```python
from build123d import *

# Parameters (mm, degrees)
SKETCH1_W           = 48.26
SKETCH1_H           = 17.78
BOSS_EXTRUDE1_DEPTH = 15.24
CUT_EXTRUDE2_DEPTH  = 18.78
BOSS_EXTRUDE2_DEPTH = 76.2
BOSS_EXTRUDE4_DEPTH = 18.21999912


with BuildPart() as part:
    # Sketch1 → Boss-Extrude1 (new body)
    with BuildSketch(Plane.XY):
        with Locations((24.13, 8.89)):
            Rectangle(SKETCH1_W, SKETCH1_H)
    extrude(amount=-BOSS_EXTRUDE1_DEPTH)

    # Sketch4 → Cut-Extrude2 (cut, through all)
    with BuildSketch(Plane(origin=(0, 17.78, 0), x_dir=(1, 0, 0), z_dir=(0, 1, 0))):
        with BuildLine():
            Line((30.48, 5.62), (22.86, 5.62))
            ThreePointArc((22.86, 5.62), (20.86, 7.62), (22.86, 9.62))
            Line((22.86, 9.62), (30.48, 9.62))
            ThreePointArc((30.48, 9.62), (32.48, 7.62), (30.48, 5.62))
        make_face()
        with BuildLine():
            Line((13.78, 5.62), (6.16, 5.62))
            ThreePointArc((6.16, 5.62), (4.16, 7.62), (6.16, 9.62))
            Line((6.16, 9.62), (13.78, 9.62))
            ThreePointArc((13.78, 9.62), (15.78, 7.62), (13.78, 5.62))
        make_face()
    extrude(amount=-CUT_EXTRUDE2_DEPTH, mode=Mode.SUBTRACT)

    # Sketch3 → Boss-Extrude2 (add)
    with BuildSketch(Plane(origin=(0, 17.78, 0), x_dir=(1, 0, 0), z_dir=(0, 1, 0))):
        Polygon((40.64, 7.62), (46.685762979, 13.665762979), (43.093660531, 13.665762979), (37.047897552, 7.62), (43.093660531, 1.574237021), (46.685762979, 1.574237021), align=None)
    extrude(amount=BOSS_EXTRUDE2_DEPTH)

    # Sketch3_7 → Boss-Extrude4 (add)
    with BuildSketch(Plane(origin=(0, 17.78, 0), x_dir=(1, 0, 0), z_dir=(0, 1, 0))):
        Polygon((48.26, 15.24), (40.64, 7.62), (48.26, 0), align=None)
    extrude(amount=BOSS_EXTRUDE4_DEPTH)


solid = part.part
```
Verification items for the finished model (mm, model axes). A direction names the side the tool comes from. Give positions to 0.01 mm unless a question says otherwise; leave off trailing zeros. Loops run counter-clockwise (first coordinate to the right, second up) from the corner with the lowest first, then second, coordinate; pieces in that order, holes last.
1. Section check A-A, the plane x = 28.5. Enter the section's corners in (y, z), then the cut area to 3 significant figures.
2. Section check B-B, the plane x = 44. Enter the section's corners in (y, z), then the cut area to 3 significant figures.
3. Thickness scan on line 1 (Z direction, x = 6.5, y = 12.5); line 2 (X direction, y = 10, z = -6); line 3 (Y direction, x = 5, z = -9.5). Record the ranges inside material, lowest first.
4. Section check D-D, the plane z = -2.5. Enter the section's corners in (x, y).
5. Set-up check for faces 4 (the flat face through (40.03, 55.35, -4.64)), 5 (the flat face through (43.71, 64.58, -4.55)), 6 (the cylindrical face through (32.48, 9.01, -7.66)), 7 (the flat face through (45, 55, -13.666)): record each of +Z, -Z, +X, -X, +Y, -Y from which the full face is reachable in a straight line by a thin tool's end or side.
6. Go/stop test with flat-tipped pins: pin 1 Ø3 at (x, y) = (45, 47.5) entering from +Z; pin 2 Ø8 at (y, z) = (50.5, -8.5) entering from +X; pin 3 Ø1 at (y, z) = (69, -8.5) entering from -X. Record where each tip stops, or that it passes through.
7. Mould release check, pull along X, two halves, no side actions. Record for faces 1 (the flat face through (24, 0, -11)), 2 (the flat face through (27, 9, -9.62)), 3 (the flat face through (43.62, 64.58, -10.6)): released by +X, released by -X, zero draft, split by the parting line, or undercut.
8. Section check C-C, the plane y = 52.5. Enter the section's corners in (x, z).
Geometry says:
1. outline: (0, -15.24) - (17.78, -15.24) - (17.78, -9.62) - (0, -9.62) - close; (0, -5.62) - (17.78, -5.62) - (17.78, 0) - (0, 0) - close
1. area: 200 mm2
2. outline: (0, -15.24) - (17.78, -15.24) - (17.78, -13.67) - (93.98, -13.67) - (93.98, -10.98) - (36, -10.98) - (36, -4.26) - (93.98, -4.26) - (93.98, -1.57) - (17.78, -1.57) - (17.78, 0) - (0, 0) - close
2. area: 803 mm2
3. line 1: z = -15.24 to -9.62, -5.62 to 0
3. line 2: x = 0 to 4.99, 14.95 to 21.69, 31.65 to 48.26
3. line 3: y = 0 to 17.78
4. outline: (0, 0) - (48.26, 0) - (48.26, 36) - (45.76, 36) - (45.76, 93.98) - (42.17, 93.98) - (42.17, 17.78) - (0, 17.78) - close
5. face 4: +Z, -X, +Y
5. face 5: +X, +Y
5. face 6: +Y, -Y
5. face 7: -Z, -X, +Y
6. pin 1: stops at z = -1.57
6. pin 2: stops at x = 45.52
6. pin 3: stops at x = 37.43
7. face 1: zero draft
7. face 2: undercut
7. face 3: released by +X
8. outline: (37.05, -7.62) - (43.09, -13.67) - (46.69, -13.67) - (40.64, -7.62) - (46.69, -1.57) - (43.09, -1.57) - close
